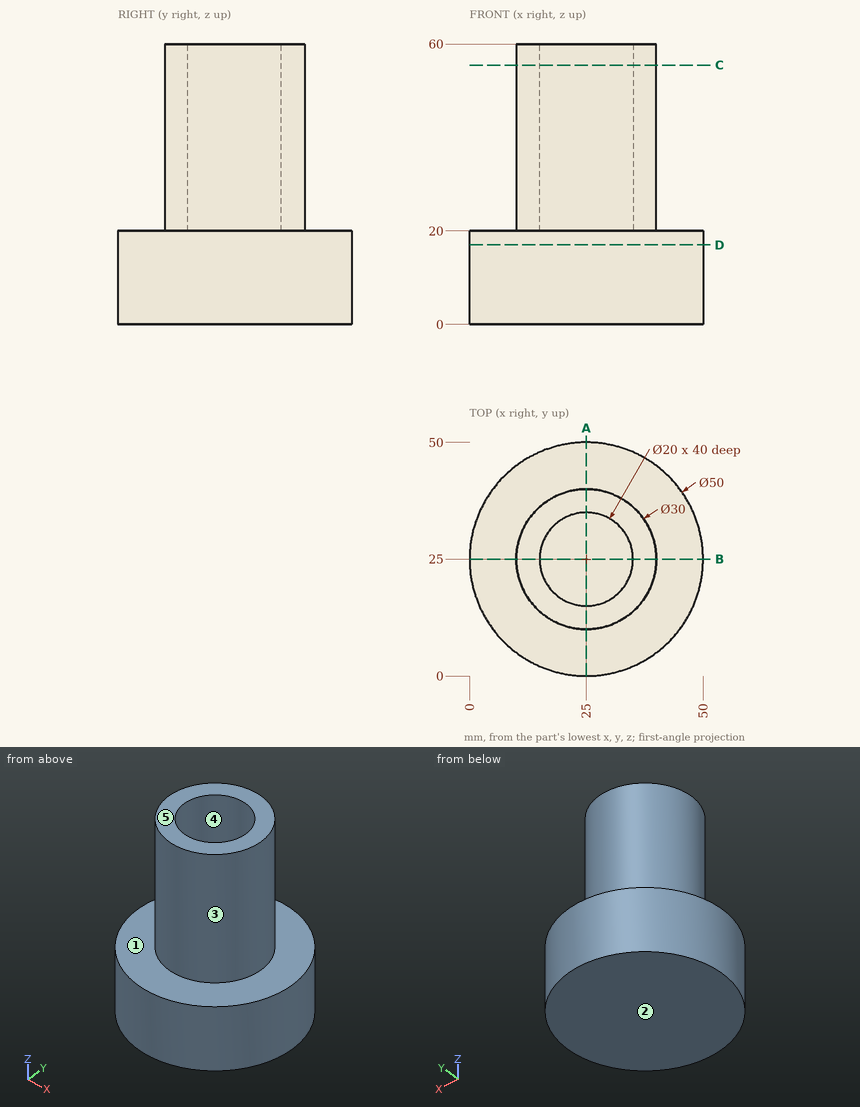
Verification items for this drawing (mm, ordinates from the low corner). A direction names the side the tool comes from. Give positions to 0.01 mm unless a question says otherwise; leave off trailing zeros. Write each loop counter-clockwise with the first axis right and the second up, starting at its lowest first coordinate (ties: lowest second). Pieces come first, ordered by that corner, then holes. Notation, with made-up numbers: (-7.5, 50) -> (38.5, 50) arc R30 cw to (38.5, 72) -> close; hole circle Ø8 at (41, -28.75). An arc over 180 degrees is marked (long way). Use CSV: the item, a comma, the result in double quotes. Start each with the question number.
Q1. Cross-section at D-D on z = 17. Enter the section's corners in (x, y), and give its area (3 significant figures).
Q2. Release check for a two-part mould opening along Y. For the marked faces 3, 4 and 5 record: +Y half, -Y half, draft (parallel to the pull), parting line (faces both ways), or undercut.
Q3. Cross-section at A-A on x = 25. Enter the section's corners in (y, z).
Q4. Depth check by flat-ended pin: P1, Ø3, axis at y = 39.5, z = 11.5, coming from the -X side; P2, Ø12, axis at y = 19, z = 52, coming from the -X side; P3, Ø8, axis at y = 25.5, z = 53, coming from the +X side. Enter the tip coordinate at first touch or a pass-through.
Q5. Cross-section at C-C on z = 55.5. Enter the section's corners in (x, y), and give its area (3 significant figures).
Q6. Scan lines: line 1 along Y through (x, z) = (25, 41); line 2 along Z through (x, y) = (22, 9.5); line 3 along X through (y, z) = (33.5, 52). Record each from-to range of solid material in increasing order.
Q7. Tool access check on the marked faces 1 and 2. Record the directions out of +Z, -Z, +X, -X, +Y, -Y that give a thin tool (end or side, any length) a straight path to the whole face; none if there is none.
Working result:
1,outline,"circle Ø50 at (25, 25)"
1,area,"1,960 mm^2"
2,face 3,"parting line"
2,face 4,"undercut"
2,face 5,"draft"
3,outline,"(0, 0) -> (50, 0) -> (50, 20) -> (40, 20) -> (40, 60) -> (35, 60) -> (35, 20) -> (15, 20) -> (15, 60) -> (10, 60) -> (10, 20) -> (0, 20) -> close"
4,P1,"stops at x = 3.65"
4,P2,"stops at x = 10"
4,P3,"stops at x = 40"
5,outline,"circle Ø30 at (25, 25); hole circle Ø20 at (25, 25)"
5,area,"393 mm^2"
6,line 1,"y = 10 to 15, 35 to 40"
6,line 2,"z = 0 to 20"
6,line 3,"x = 12.64 to 19.73, 30.27 to 37.36"
7,face 1,"+Z"
7,face 2,"-Z, +X, -X, +Y, -Y"
